Job drawing, mm, ordinate dimensions from the low corner. One solid piece. A direction names the side the tool comes from. Round coordinates to 2 decimals unless told otherwise and drop trailing zeros. Write each loop counter-clockwise with the first axis right and the second up, starting at its lowest first coordinate (ties: lowest second). Pieces come first, ordered by that corner, then holes.
1) Flat gauge pins, fed straight in: pin 1 (5 mm diameter, centred on x = 15.5, y = 8.5, fed in from -Z); pin 2 (10 mm diameter, centred on x = 14, z = 13.5, fed in from +Y); pin 3 (4 mm diameter, centred on x = 15.5, z = 8.5, fed in from +Y); pin 4 (7 mm diameter, centred on x = 20.5, y = 9, fed in from +Z). Where does each tip first touch, or does it go through?
2) Saw through at B-B on z = 8.5. Write the cut outline in (x, y).
3) Saw through at A-A on x = 31.5. Write the cut outline in (y, z), and give its area (3 significant figures).
4) Saw through at D-D on x = 11.5. Write the cut outline in (y, z), and give its area (3 significant figures).
5) Which spindle directions (+Z, -Z, +X, -X, +Y, -Y) get a long thin tool onto all of the face, cutting with end or side? Do the marked faces 1 and 2. Say none if no direction does.
6) Saw through at C-C on y = 8.2. Write the cut outline in (x, z).
7) Drill centre lines: L1, parallel to X at y = 0.85, z = 8.5; L2, parallel to Z at x = 15.5, y = 1.1 (3 decimals); L3, parallel to Z at x = 13, y = 11. Where is each one in solid material? Low to high.
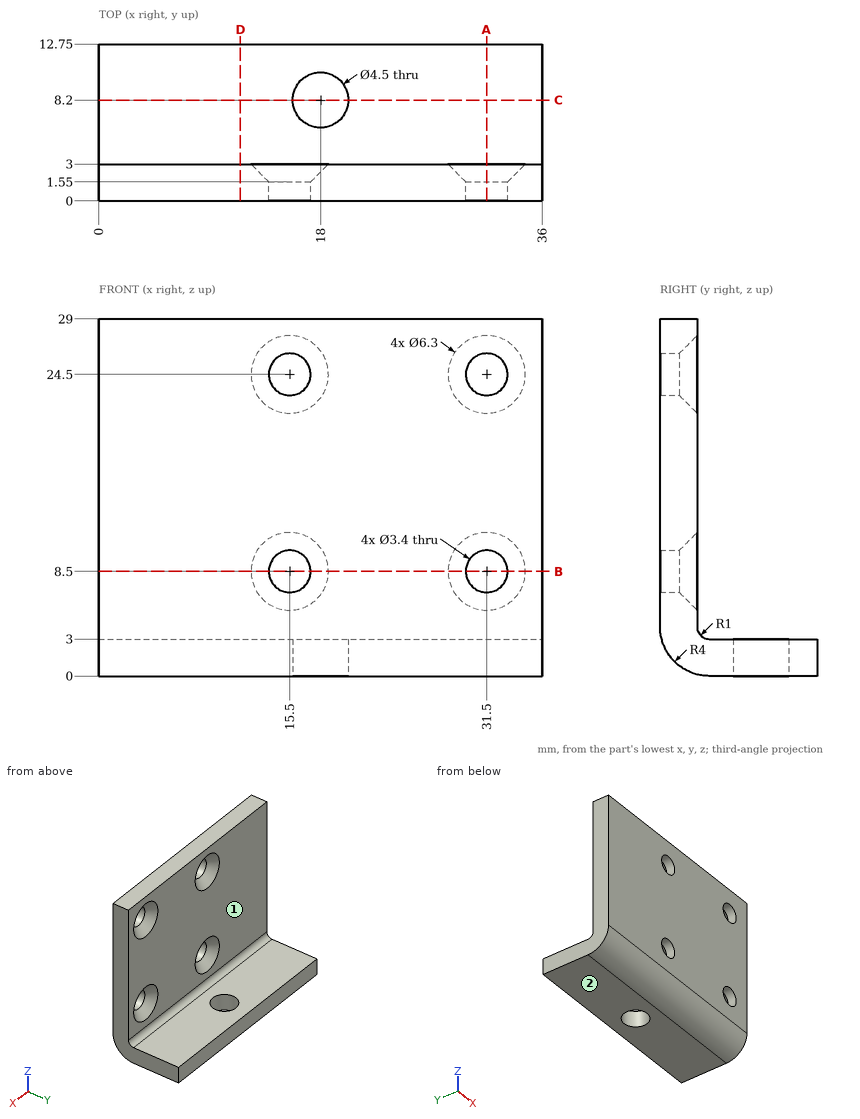
Completed:
1. pin 1: stops at z = 0
1. pin 2: stops at y = 3
1. pin 3: stops at y = 1.85
1. pin 4: stops at z = 3
2. outline: (0, 0) - (13.8, 0) - (13.8, 1.55) - (12.35, 3) - (0, 3) - close; (17.2, 0) - (29.8, 0) - (29.8, 1.55) - (28.35, 3) - (18.65, 3) - (17.2, 1.55) - close; (33.2, 0) - (36, 0) - (36, 3) - (34.65, 3) - (33.2, 1.55) - close
3. outline: (0, 4) arc R4 ccw to (4, 0) - (12.75, 0) - (12.75, 3) - (4, 3) arc R1 cw to (3, 4) - (3, 5.35) - (1.55, 6.8) - (0, 6.8) - close; (0, 10.2) - (1.55, 10.2) - (3, 11.65) - (3, 21.35) - (1.55, 22.8) - (0, 22.8) - close; (0, 26.2) - (1.55, 26.2) - (3, 27.65) - (3, 29) - (0, 29) - close
3. area: 88.4 mm2
4. outline: (0, 4) arc R4 ccw to (4, 0) - (12.75, 0) - (12.75, 3) - (4, 3) arc R1 cw to (3, 4) - (3, 29) - (0, 29) - close
4. area: 113 mm2
5. face 1: +Z, +X, -X, +Y
5. face 2: -Z, +X, -X, +Y, -Y
6. outline: (0, 0) - (15.75, 0) - (15.75, 3) - (0, 3) - close; (20.25, 0) - (36, 0) - (36, 3) - (20.25, 3) - close
7. L1: x = 0 to 13.8, 17.2 to 29.8, 33.2 to 36
7. L2: z = 1.245 to 6.8, 10.2 to 22.8, 26.2 to 29
7. L3: z = 0 to 3
